Could you check a few things on this model? Use its own coordinates, in mm. Face numbers are marked on the shaded views. A direction names the side the tool comes from. Round coordinates to 2 decimals unless told otherwise and drop trailing zeros. Write each loop counter-clockwise with the first axis right and the second up, starting at its lowest first coordinate (ties: lowest second). Pieces come first, ordered by that corner, then holes. Notation, with made-up numbers: (-2.75, -1.75) - (4.25, -1.75) arc R20 cw to (4.25, 22.25) - close; hole circle Ø2 at (61.25, 56). An arc over 180 degrees is marked (long way). Put each result on its own line as item: value.
from build123d import *

# Parameters (mm, degrees)
F0_R     = 11.8
F1_DEPTH = 1.25
F3_DEPTH = 2.501
F5_DEPTH = 2.501


with BuildPart() as f1:
    # F0 (on Front) → F1 (new body, symmetric)
    with BuildSketch(Plane.XZ):
        Circle(F0_R)
    extrude(amount=F1_DEPTH, both=True)

    # F2 (on face) → F3 (cut, through all)
    with BuildSketch(Plane(origin=(0, 1.25, 0), x_dir=(-1, 0, 0), z_dir=(0, 1, 0))):
        with BuildLine():
            ThreePointArc((0, 10.8), (-0.794118, 10.770765), (-1.583936, 10.683218))
            Line((-1.583936, 10.683218), (-0.997293, 6.726471))
            ThreePointArc((-0.997293, 6.726471), (-0.5, 6.781593), (0, 6.8))
            Line((0, 6.8), (0, 10.8))
        make_face()
        with BuildLine():
            ThreePointArc((-6.371006, 8.673176), (-6.996277, 8.182754), (-7.583795, 7.647683))
            Line((-7.583795, 7.647683), (-4.783473, 4.791428))
            ThreePointArc((-4.783473, 4.791428), (-4.413554, 5.128324), (-4.019865, 5.437108))
            Line((-4.019865, 5.437108), (-6.371006, 8.673176))
        make_face()
        with BuildLine():
            ThreePointArc((-8.755893, 6.249643), (-9.199012, 5.590005), (-9.592429, 4.899569))
            Line((-9.592429, 4.899569), (-6.046533, 3.048456))
            ThreePointArc((-6.046533, 3.048456), (-5.798826, 3.483174), (-5.519825, 3.898502))
            Line((-5.519825, 3.898502), (-8.755893, 6.249643))
        make_face()
        with BuildLine():
            ThreePointArc((-10.275143, 3.207756), (-10.492735, 2.443471), (-10.65354, 1.665256))
            Line((-10.65354, 1.665256), (-6.709167, 1.000484))
            ThreePointArc((-6.709167, 1.000484), (-6.607919, 1.490472), (-6.470917, 1.971688))
            Line((-6.470917, 1.971688), (-10.275143, 3.207756))
        make_face()
        with BuildLine():
            ThreePointArc((-10.78004, -0.154725), (-10.750805, -0.948842), (-10.663258, -1.738661))
            Line((-10.663258, -1.738661), (-6.706511, -1.152018))
            ThreePointArc((-6.706511, -1.152018), (-6.761633, -0.654725), (-6.78004, -0.154725))
            Line((-6.78004, -0.154725), (-10.78004, -0.154725))
        make_face()
        with BuildLine():
            ThreePointArc((-10.221163, -3.508656), (-9.947962, -4.254872), (-9.620633, -4.978981))
            Line((-9.620633, -4.978981), (-6.038825, -3.198348))
            ThreePointArc((-6.038825, -3.198348), (-6.244922, -2.742428), (-6.416936, -2.272588))
            Line((-6.416936, -2.272588), (-10.221163, -3.508656))
        make_face()
        with BuildLine():
            ThreePointArc((-8.653216, -6.525731), (-8.162794, -7.151002), (-7.627724, -7.738519))
            Line((-7.627724, -7.738519), (-4.771468, -4.938197))
            ThreePointArc((-4.771468, -4.938197), (-5.108364, -4.568279), (-5.417149, -4.17459))
            Line((-5.417149, -4.17459), (-8.653216, -6.525731))
        make_face()
        with BuildLine():
            ThreePointArc((-6.229684, -8.910618), (-5.570045, -9.353737), (-4.87961, -9.747154))
            Line((-4.87961, -9.747154), (-3.028496, -6.201258))
            ThreePointArc((-3.028496, -6.201258), (-3.463215, -5.953551), (-3.878543, -5.67455))
            Line((-3.878543, -5.67455), (-6.229684, -8.910618))
        make_face()
        with BuildLine():
            ThreePointArc((-3.187796, -10.429868), (-2.423511, -10.647459), (-1.645296, -10.808264))
            Line((-1.645296, -10.808264), (-0.980524, -6.863891))
            ThreePointArc((-0.980524, -6.863891), (-1.470512, -6.762644), (-1.951728, -6.625641))
            Line((-1.951728, -6.625641), (-3.187796, -10.429868))
        make_face()
        with BuildLine():
            ThreePointArc((0.174684, -10.934765), (0.968802, -10.90553), (1.75862, -10.817983))
            Line((1.75862, -10.817983), (1.171977, -6.861235))
            ThreePointArc((1.171977, -6.861235), (0.674684, -6.916358), (0.174684, -6.934765))
            Line((0.174684, -6.934765), (0.174684, -10.934765))
        make_face()
        with BuildLine():
            ThreePointArc((3.528615, -10.375887), (4.274832, -10.102687), (4.99894, -9.775358))
            Line((4.99894, -9.775358), (3.218308, -6.19355))
            ThreePointArc((3.218308, -6.19355), (2.762387, -6.399646), (2.292547, -6.571661))
            Line((2.292547, -6.571661), (3.528615, -10.375887))
        make_face()
        with BuildLine():
            ThreePointArc((6.545691, -8.807941), (7.170961, -8.317519), (7.758479, -7.782448))
            Line((7.758479, -7.782448), (4.958157, -4.926192))
            ThreePointArc((4.958157, -4.926192), (4.588239, -5.263089), (4.19455, -5.571873))
            Line((4.19455, -5.571873), (6.545691, -8.807941))
        make_face()
        with BuildLine():
            ThreePointArc((8.930578, -6.384408), (9.373697, -5.72477), (9.767113, -5.034334))
            Line((9.767113, -5.034334), (6.221217, -3.183221))
            ThreePointArc((6.221217, -3.183221), (5.973511, -3.617939), (5.69451, -4.033267))
            Line((5.69451, -4.033267), (8.930578, -6.384408))
        make_face()
        with BuildLine():
            ThreePointArc((10.449827, -3.342521), (10.667419, -2.578236), (10.828224, -1.800021))
            Line((10.828224, -1.800021), (6.883851, -1.135249))
            ThreePointArc((6.883851, -1.135249), (6.782603, -1.625237), (6.645601, -2.106453))
            Line((6.645601, -2.106453), (10.449827, -3.342521))
        make_face()
        with BuildLine():
            ThreePointArc((10.954725, 0.01996), (10.92549, 0.814077), (10.837943, 1.603896))
            Line((10.837943, 1.603896), (6.881195, 1.017253))
            ThreePointArc((6.881195, 1.017253), (6.936317, 0.51996), (6.954725, 0.01996))
            Line((6.954725, 0.01996), (10.954725, 0.01996))
        make_face()
        with BuildLine():
            ThreePointArc((10.395847, 3.373891), (10.122647, 4.120107), (9.795317, 4.844216))
            Line((9.795317, 4.844216), (6.21351, 3.063583))
            ThreePointArc((6.21351, 3.063583), (6.419606, 2.607663), (6.591621, 2.137823))
            Line((6.591621, 2.137823), (10.395847, 3.373891))
        make_face()
        with BuildLine():
            ThreePointArc((8.827901, 6.390966), (8.337478, 7.016237), (7.802408, 7.603754))
            Line((7.802408, 7.603754), (4.946152, 4.803432))
            ThreePointArc((4.946152, 4.803432), (5.283048, 4.433514), (5.591833, 4.039825))
            Line((5.591833, 4.039825), (8.827901, 6.390966))
        make_face()
        with BuildLine():
            ThreePointArc((6.404368, 8.775853), (5.744729, 9.218972), (5.054294, 9.612389))
            Line((5.054294, 9.612389), (3.20318, 6.066493))
            ThreePointArc((3.20318, 6.066493), (3.637899, 5.818786), (4.053227, 5.539785))
            Line((4.053227, 5.539785), (6.404368, 8.775853))
        make_face()
        with BuildLine():
            ThreePointArc((3.362481, 10.295103), (2.598196, 10.512694), (1.81998, 10.6735))
            Line((1.81998, 10.6735), (1.155209, 6.729126))
            ThreePointArc((1.155209, 6.729126), (1.645196, 6.627879), (2.126413, 6.490877))
            Line((2.126413, 6.490877), (3.362481, 10.295103))
        make_face()
        with BuildLine():
            ThreePointArc((-3.353931, 10.241122), (-4.100148, 9.967922), (-4.824256, 9.640593))
            Line((-4.824256, 9.640593), (-3.043623, 6.058785))
            ThreePointArc((-3.043623, 6.058785), (-2.587703, 6.264881), (-2.117863, 6.436896))
            Line((-2.117863, 6.436896), (-3.353931, 10.241122))
        make_face()
    extrude(amount=-F3_DEPTH, mode=Mode.SUBTRACT)

    # F4 (on face) → F5 (cut, through all)
    with BuildSketch(Plane(origin=(0, 1.25, 0), x_dir=(-1, 0, 0), z_dir=(0, 1, 0))):
        with BuildLine():
            Line((-1.75, 2.12132), (-1.75, -2.12132))
            ThreePointArc((-1.75, -2.12132), (0, -2.75), (1.75, -2.12132))
            Line((1.75, -2.12132), (1.75, 2.12132))
            ThreePointArc((1.75, 2.12132), (0, 2.75), (-1.75, 2.12132))
        make_face()
    extrude(amount=-F5_DEPTH, mode=Mode.SUBTRACT)


solid = f1.part
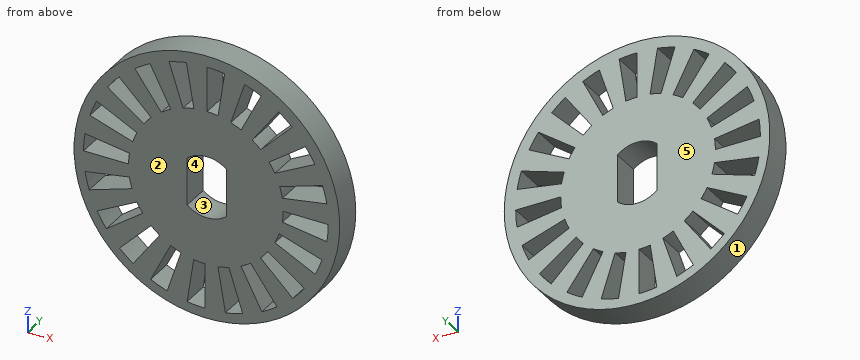
(1) Imagine slicing it at A-A, the plane x = 2.5. List the corners of the cut face in (y, z) for me.
Values found:
outline: (-1.25, -11.53) - (1.25, -11.53) - (1.25, -10.63) - (-1.25, -10.63) - close; (-1.25, -8.31) - (1.25, -8.31) - (1.25, 6.3) - (-1.25, 6.3) - close; (-1.25, 7.61) - (1.25, 7.61) - (1.25, 11.53) - (-1.25, 11.53) - close
(2) Imagine slicing it at B-B, the plane z = -0.5. List the corners of the cut face in (x, y) for me.
Values found:
outline: (-11.79, -1.25) - (-1.75, -1.25) - (-1.75, 1.25) - (-11.79, 1.25) - close; (1.75, -1.25) - (6.77, -1.25) - (6.77, 1.25) - (1.75, 1.25) - close; (10.77, -1.25) - (11.79, -1.25) - (11.79, 1.25) - (10.77, 1.25) - close
(3) I'm going to push flat-ended pins straight in: pin 1 (1.2 mm diameter, centred on x = 9, y = 0, fed in from -Z); pin 2 (0.8 mm diameter, centred on y = 0, z = -9, fed in from -X); pin 3 (1.2 mm diameter, centred on y = -0.5, z = 8, fed in from +X). Where does each tip first touch, or does it pass through?
Values found:
pin 1: stops at z = -8.29
pin 2: stops at x = -8.08
pin 3: stops at x = 9.19
(4) If we mould it in two halves opening along Z, with no side actions, what happens to the marked faces 1, 2 and 3? For each: pulls with the +Z half, pulls with the -Z half, needs draft (parallel to the pull), parting line crosses it, or undercut.
Values found:
face 1: parting line crosses it
face 2: needs draft
face 3: undercut
(5) Imagine slicing it at C-C, the plane y = -0.8. Give the number of separate pieces and of enclosed holes in the cut face, then the cut area to 3 significant figures.
Values found:
separate pieces: 1
enclosed holes: 21
area: 316 mm^2
(6) Please list where these lines run through material, in increasing order: probe 1 along X at (y, z) = (-0.3, 5); probe 2 along X at (y, z) = (-1.05, 0.5); probe 3 along X at (y, z) = (0.4, -2). Write a range as from..to.
Values found:
probe 1: x = -10.69..-6.91, -5.15..4.56, 4.99..7.04, 9.54..10.69
probe 2: x = -11.79..-10.94, -6.94..-1.75, 1.75..11.79
probe 3: x = -11.63..-10.79, -6.68..-1.75, 1.75..11.63
(7) For the marked faces 4 and 5, which set-ups out of +Z, -Z, +X, -X, +Y, -Y let a thin tool reach every point of the face, with its end or its side?
Values found:
face 4: +Y, -Y
face 5: +Z, -Z, +X, -X, +Y
